Work out the finished part from the listing and answer in its coordinate system (mm). A direction names the side the tool comes from. Coordinates: 2 decimals unless noted, no trailing zeros. Loops run counter-clockwise (first coordinate to the right, second up) from the corner with the lowest first, then second, coordinate; pieces in that order, holes last.
```python
from build123d import *

# Parameters (mm, degrees)
F0_R     = 1.5
F1_DEPTH = 4.5
F2_R     = 1.5
F3_DEPTH = 20.001
F4_R     = 4


with BuildPart() as f1:
    # F0 (on Top) → F1 (new body, symmetric)
    with BuildSketch(Plane.XY):
        Polygon((-5, 17.5), (-10, 17.5), (-10, -6.5), (-4.5, -6.5), (-4.5, -17.5), (4.5, -17.5), (4.5, -6.5), (10, -6.5), (10, 17.5), (5, 17.5), (5, 6.5), (-5, 6.5), align=None)
        with Locations((0, -12.5)):
            Circle(F0_R, mode=Mode.SUBTRACT)
    extrude(amount=F1_DEPTH, both=True)

    # F2 (on face) → F3 (cut, through all)
    with BuildSketch(Plane.YZ.offset(10)):
        with Locations((12.5, 0)):
            Circle(F2_R)
    extrude(amount=-F3_DEPTH, mode=Mode.SUBTRACT)

    # F4
    f4_edges = [f1.edges().sort_by_distance(p)[0] for p in [
        (4.5, -17.5, 0),
        (-4.5, -17.5, 0),
        (7.5, 17.5, 4.5),
        (7.5, 17.5, -4.5),
        (-7.5, 17.5, -4.5),
        (-7.5, 17.5, 4.5),
        (10, -6.5, 0),
        (-10, -6.5, 0),
    ]]
    fillet(f4_edges, radius=F4_R)


solid = f1.part
```
1. A cutting plane is placed at A-A, the plane z = 0. Give the vertices of the cut face in (x, y).
2. Determine the mould class of faces 4 (the flat face through (-4.5, -10, 0)), 5 (the cylindrical face through (8, 11, 0)), 6 (the flat face through (0, -2, 4.5)), 7 (the flat face through (0, -2, -4.5)) for opening direction Z: released by +Z, released by -Z, zero draft, split by the parting line, or undercut.
3. A cutting plane is placed at D-D, the plane x = 0. Give the vertices of the cut face in (y, z), then the cut area to 3 significant figures.
4. A cutting plane is placed at B-B, the plane y = 12.5. Give the vertices of the cut face in (x, z), then the cut area to 3 significant figures.
5. For faces 1 (the flat face through (4.5, -10, 0)), 2 (the flat face through (10, 7, 0)), 3 (the flat face through (-5, 10.7, 0.1)), determine the directions among +Z, -Z, +X, -X, +Y, -Y from which every point of the face is accessible in a straight line to the end or side of a thin tool.
6. Each of these flat-tipped pins is pushed along its axis until it touches: P1, Ø2.5, axis at y = 12.5, z = 0, coming from the -X side (3 decimals); P2, Ø0.5, axis at x = 5.5, z = 0.5, coming from the -Y side; P3, Ø1.5, axis at x = -1.5, z = -3, coming from the -Y side; P4, Ø3, axis at x = 3.5, z = 1.5, coming from the -Y side. Where does it stop, or does it pass through?
7. A cutting plane is placed at C-C, the plane y = -12.5. Give the vertices of the cut face in (x, z).
8. Straight lines are drawn through the part: probe 1 along X at (y, z) = (13, 3.5); probe 2 along Z at (x, y) = (8.25, 12.5); probe 3 along Y at (x, z) = (0, -1.25). For each, find the intervals that lie inside material, in ascending order.
Answers below:
1. outline: (-10, -2.5) arc R4 ccw to (-6, -6.5) - (-4.5, -6.5) - (-4.5, -13.5) arc R4 ccw to (-0.5, -17.5) - (0.5, -17.5) arc R4 ccw to (4.5, -13.5) - (4.5, -6.5) - (6, -6.5) arc R4 ccw to (10, -2.5) - (10, 11) - (5, 11) - (5, 6.5) - (-5, 6.5) - (-5, 11) - (-10, 11) - close; (-10, 14) - (-5, 14) - (-5, 17.5) - (-10, 17.5) - close; (5, 14) - (10, 14) - (10, 17.5) - (5, 17.5) - close; hole circle Ø3 at (0, -12.5)
2. face 4: zero draft
2. face 5: undercut
2. face 6: released by +Z
2. face 7: released by -Z
3. outline: (-17.5, -4.5) - (-14, -4.5) - (-14, 4.5) - (-17.5, 4.5) - close; (-11, -4.5) - (6.5, -4.5) - (6.5, 4.5) - (-11, 4.5) - close
3. area: 189 mm2
4. outline: (-10, -4.5) - (-5, -4.5) - (-5, -1.5) - (-10, -1.5) - close; (-10, 1.5) - (-5, 1.5) - (-5, 4.5) - (-10, 4.5) - close; (5, -4.5) - (10, -4.5) - (10, -1.5) - (5, -1.5) - close; (5, 1.5) - (10, 1.5) - (10, 4.5) - (5, 4.5) - close
4. area: 60.0 mm2
5. face 1: +Z, -Z, +X, -Y
5. face 2: +Z, -Z, +X, +Y, -Y
5. face 3: +Z, -Z, +Y
6. P1: passes through
6. P2: stops at y = -6.5
6. P3: stops at y = -17.49
6. P4: stops at y = -17.21
7. outline: (-4.5, -4.5) - (-1.5, -4.5) - (-1.5, 4.5) - (-4.5, 4.5) - close; (1.5, -4.5) - (4.5, -4.5) - (4.5, 4.5) - (1.5, 4.5) - close
8. probe 1: x = -10 to -5, 5 to 10
8. probe 2: z = -4.5 to -1.5, 1.5 to 4.5
8. probe 3: y = -17.5 to -14, -11 to 6.5
